from build123d import *

# Parameters (mm, degrees)
SKETCH_2_W               = 29.4
SKETCH_2_H               = 25
EXTRUDE_1_DEPTH          = 8
CUT_EXTRUDE_1_DEPTH      = 31.58578101
CUT_EXTRUDE_1_DEPTH_BACK = 31.58578101
SKETCH_3_R               = 1.35


with BuildPart() as part:
    # 草图2 → 凸台-拉伸1 (new body)
    with BuildSketch(Plane.XY):
        with Locations((1, -1.6)):
            Rectangle(SKETCH_2_W, SKETCH_2_H)
        with BuildLine():
            ThreePointArc((8.2, -7.2), (8.053553391, -7.553553391), (7.7, -7.7))
            Line((7.7, -7.7), (-7.7, -7.7))
            ThreePointArc((-7.7, -7.7), (-8.2, -7.2), (-7.7, -6.7))
            Line((-7.7, -6.7), (-7.7, 6.7))
            ThreePointArc((-7.7, 6.7), (-8.2, 7.2), (-7.7, 7.7))
            Line((-7.7, 7.7), (7.7, 7.7))
            ThreePointArc((7.7, 7.7), (8.053553391, 7.553553391), (8.2, 7.2))
            ThreePointArc((8.2, 7.2), (8.053553391, 6.846446609), (7.7, 6.7))
            Line((7.7, 6.7), (7.7, -6.7))
            ThreePointArc((7.7, -6.7), (8.053553391, -6.846446609), (8.2, -7.2))
        make_face(mode=Mode.SUBTRACT)
    extrude(amount=EXTRUDE_1_DEPTH)

    # 草图3 → 切除-拉伸1 (cut, two sides: drawn at the far end of the back side and taken through both)
    with BuildSketch(Plane(origin=(0, 10.9, 0), x_dir=(1, 0, 0), z_dir=(0, 1, 0)).offset(-CUT_EXTRUDE_1_DEPTH_BACK)):
        with Locations(Location((10.5, -4, 0), (0, 0, 270))):
            Circle(SKETCH_3_R)
        with Locations((21, -4)):
            Circle(SKETCH_3_R)
        with Locations(Location((0, -4, 0), (0, 0, 270))):
            Circle(SKETCH_3_R)
    extrude(amount=CUT_EXTRUDE_1_DEPTH + CUT_EXTRUDE_1_DEPTH_BACK, mode=Mode.SUBTRACT)


solid = part.part
Source: CAD feature listing. Evaluate the final solid. Frame: model axes, mm. A direction names the side the tool comes from. Coordinates: 2 decimals unless noted, no trailing zeros. Loops run counter-clockwise (first coordinate to the right, second up) from the corner with the lowest first, then second, coordinate; pieces in that order, holes last. Notation, with made-up numbers: (-40, 35.5) -> (-19, 35.5) arc R29 cw to (-19, 69.5) -> close; hole circle Ø5 at (66.5, 82.25). An arc over 180 degrees is marked (long way). Answer in a Markdown table with one row per item. Add a question column.
Q1. Section B-B on x = 3. Return the cut outline in (y, z).
Q2. Section D-D on x = 10.5. Return the cut outline in (y, z).
Q3. Ray query, line 1 along X through (y, z) = (9, 4); line 2 along Y through (x, z) = (7.75, 2.75); line 3 along Y through (x, z) = (6, 6.5). Return the intervals inside material, ascending.
Q4. Section C-C on z = 4. Return the cut outline in (x, y).
Q5. Section A-A on y = 1.25. Return the cut outline in (x, z).
Q6. Pull-direction query (X, two-part tool) for faces 3 (the face through (1, -10, 8)), 4 (the face through (2, -7.7, 4)), 5 (the face through (15.7, -2, 4)); classes: pulls with the +X half, pulls with the -X half, needs draft (parallel to the pull), parting line crosses it, or undercut.
Q7. Reachability of faces 1 (the face through (-13.7, -2, 4)), 2 (the face through (-8.2, 7.2, 3.9)) from +Z, -Z, +X, -X, +Y, -Y: full face, straight path, thin tool, end or side. Return the list, or none.
Computed values:
| question | item | result |
|---|---|---|
| 1 | outline | (-14.1, 0) -> (-7.7, 0) -> (-7.7, 8) -> (-14.1, 8) -> close; (7.7, 0) -> (10.9, 0) -> (10.9, 8) -> (7.7, 8) -> close |
| 2 | outline | (-14.1, 0) -> (10.9, 0) -> (10.9, 2.65) -> (-14.1, 2.65) -> close; (-14.1, 5.35) -> (10.9, 5.35) -> (10.9, 8) -> (-14.1, 8) -> close |
| 3 | line 1 | x = -13.7 to -1.35, 1.35 to 9.15, 11.85 to 15.7 |
| 3 | line 2 | y = -14.1 to -7.7, -6.7 to 6.7, 7.7 to 10.9 |
| 3 | line 3 | y = -14.1 to -7.7, 7.7 to 10.9 |
| 4 | outline | (-13.7, -14.1) -> (-1.35, -14.1) -> (-1.35, -7.7) -> (-7.7, -7.7) arc R0.5 cw to (-7.7, -6.7) -> (-7.7, 6.7) arc R0.5 cw to (-7.7, 7.7) -> (-1.35, 7.7) -> (-1.35, 10.9) -> (-13.7, 10.9) -> close; (1.35, -14.1) -> (9.15, -14.1) -> (9.15, 10.9) -> (1.35, 10.9) -> (1.35, 7.7) -> (7.7, 7.7) arc R0.5 cw to (7.7, 6.7) -> (7.7, -6.7) arc R0.5 cw to (7.7, -7.7) -> (1.35, -7.7) -> close; (11.85, -14.1) -> (15.7, -14.1) -> (15.7, 10.9) -> (11.85, 10.9) -> close |
| 5 | outline | (-13.7, 0) -> (-7.7, 0) -> (-7.7, 8) -> (-13.7, 8) -> close; (7.7, 0) -> (15.7, 0) -> (15.7, 8) -> (7.7, 8) -> close; hole circle Ø2.7 at (10.5, 4) |
| 6 | face 3 | needs draft |
| 6 | face 4 | undercut |
| 6 | face 5 | pulls with the +X half |
| 7 | face 1 | +Z, -Z, -X, +Y, -Y |
| 7 | face 2 | +Z, -Z |
